Part model, mm, in its own coordinate system. Face numbers are marked on the shaded views. A direction names the side the tool comes from. Give positions to 0.01 mm unless a question says otherwise; leave off trailing zeros. Write each loop counter-clockwise with the first axis right and the second up, starting at its lowest first coordinate (ties: lowest second). Pieces come first, ordered by that corner, then holes.
Autodesk Inventor part; units mm, degrees
ref_plane "YZ Plane" through (0, 0, 0) normal (1, 0, 0) x (0, 1, 0)
ref_plane "XZ Plane" through (0, 0, 0) normal (0, 1, 0) x (-1, 0, 0)
ref_plane "XY Plane" through (0, 0, 0) normal (0, 0, 1) x (1, 0, 0)
sketch "Boceto1" plane through (0, 0, 0) normal (0, 1, 0) x (-1, 0, 0)
  line L0 (26.75, 89.25) -> (-26.75, 89.25)
  line L1 (-26.75, 89.25) -> (-26.75, -89.25)
  line L2 (-26.75, -89.25) -> (26.75, -89.25)
  line L3 (26.75, -89.25) -> (26.75, 89.25)
  line L4 (26.75, 89.25) -> (-26.75, -89.25) construction
  line L5 (-26.75, 89.25) -> (26.75, -89.25) construction
  point P0 (0, 0)
  dimension "d0" = 53.5
  dimension "d1" = 178.5
extrude "Extrusión1" add sketch "Boceto1" along normal blind 50
sketch "Boceto2" plane through (0, 50, 0) normal (0, 1, 0) x (1, 0, 0)
  line L0 (-25.5, -88) -> (25.5, -88)
  line L1 (25.5, -88) -> (25.5, 88)
  line L2 (25.5, 88) -> (-25.5, 88)
  line L3 (-25.5, 88) -> (-25.5, -88)
  line L4 (-25.5, -88) -> (25.5, 88) construction
  line L5 (25.5, -88) -> (-25.5, 88) construction
  point P0 (0, 0)
  dimension "d4" = 51
  dimension "d5" = 176
extrude "Extrusión2" cut sketch "Boceto2" against normal blind 47.5
sketch "Boceto3" plane through (26.75, 0, 89.25) normal (1, 0, 0) x (0, 0, -1)
  line L0 (52.25, 50) -> (52.25, 20)
  line L1 (0, 0) -> (178.5, 0)
  line L2 (126.25, 50) -> (126.25, 20)
  line L3 (126.25, 20) -> (52.25, 20)
  line L4 (52.25, 50) -> (126.25, 50)
  point P0 (89.25, 0)
  point P1 (177.25, 50)
  point P2 (1.25, 50)
  dimension "d9" = 30
extrude "Extrusión3" cut sketch "Boceto3" against normal through all
properties part number "Suport motor superior" material "Plástico ABS"
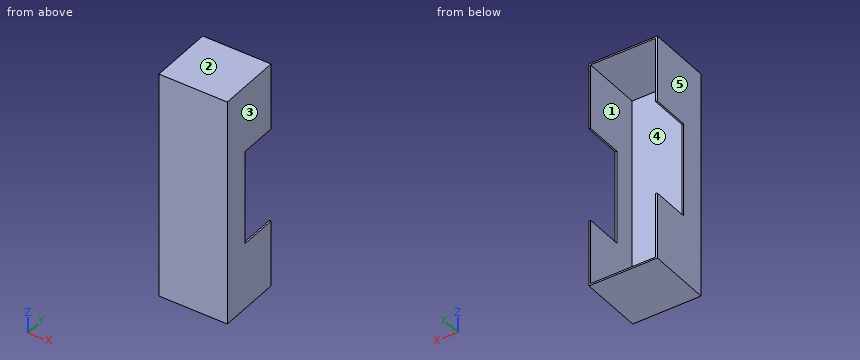
1) Drill centre lines: L1, parallel to Z at x = -7.5, y = 35; L2, parallel to X at y = 32.5, z = 51.5; L3, parallel to Y at x = -12.5, z = 38. Where is each one in solid material? Low to high.
Check result:
L1: z = -89.25 to -88, 88 to 89.25
L2: x = -26.75 to -25.5, 25.5 to 26.75
L3: y = 0 to 2.5
2) Flat gauge pins, fed straight in: P1, Ø12, axis at x = -10, z = 7.5, coming from the +Y side; P2, Ø1, axis at x = 26, z = -5, coming from the +Y side. Where does each tip first touch, or does it go through?
Check result:
P1: stops at y = 2.5
P2: stops at y = 20
3) Saw through at A-A (y = 29). Write the cut outline in (x, z).
Check result:
outline: (-26.75, -89.25) - (26.75, -89.25) - (26.75, -37) - (25.5, -37) - (25.5, -88) - (-25.5, -88) - (-25.5, -37) - (-26.75, -37) - close; (-26.75, 37) - (-25.5, 37) - (-25.5, 88) - (25.5, 88) - (25.5, 37) - (26.75, 37) - (26.75, 89.25) - (-26.75, 89.25) - close
4) 3-axis set-ups, long thin cutter, end or side, ignore diameter. For the marked faces 1 and 2: which of +Z, -Z, +X, -X, +Y, -Y reach the whole face in a straight line?
Check result:
face 1: +Y
face 2: +Z, +X, -X, +Y, -Y
5) Saw through at D-D (y = 12). Write the cut outline in (x, z), and give its area (3 significant figures).
Check result:
outline: (-26.75, -89.25) - (26.75, -89.25) - (26.75, 89.25) - (-26.75, 89.25) - close; hole (-25.5, -88) - (25.5, -88) - (25.5, 88) - (-25.5, 88) - close
area: 574 mm2
6) Saw through at B-B (x = 9). Write the cut outline in (y, z).
Check result:
outline: (0, -89.25) - (50, -89.25) - (50, -88) - (2.5, -88) - (2.5, 88) - (50, 88) - (50, 89.25) - (0, 89.25) - close
7) Mould opens along X. For the marked faces 3, 4 and 5 say: +X half, -X half, draft (parallel to the pull), parting line (faces both ways), or undercut.
Check result:
face 3: +X half
face 4: undercut
face 5: -X half
8) Saw through at C-C (z = -13.5). Write the cut outline in (x, y), and give its area (4 significant figures).
Check result:
outline: (-26.75, 0) - (26.75, 0) - (26.75, 20) - (25.5, 20) - (25.5, 2.5) - (-25.5, 2.5) - (-25.5, 20) - (-26.75, 20) - close
area: 177.5 mm2
